Part model, mm, in its own coordinate system. A direction names the side the tool comes from. Coordinates: 2 decimals unless noted, no trailing zeros. Write each loop counter-clockwise with the first axis right and the second up, starting at its lowest first coordinate (ties: lowest second). Pieces come first, ordered by that corner, then holes. Notation, with made-up numbers: (0, 32) -> (36, 32) arc R22 cw to (36, 70) -> close; hole circle Ø9 at (-1.5, 60.25). An arc over 180 degrees is marked (long way). Write item = value, one per line. Start each with the question number.
Q1. Band-saw the part on C-C, the plane y = -6. List the corners of the cut face in (x, z), plus the area to 3 significant figures.
Q2. Tool access for faces 1 (the cylindrical face through (-1, -2, 65)), 2 (the flat face through (12, -10, 30)), 3 (the cylindrical face through (-1, -2, 15)), 4 (the cylindrical face through (13, -18, 31)): list every direction of +Z, -Z, +X, -X, +Y, -Y with a clear straight run to the whole face (end or side of a thin tool).
Q3. Pull direction Y, two halves, no side cores. Call faces 5 (the cylindrical face through (24, -18, 40)), 6 (the cylindrical face through (10, -10, 41)), 7 (the cylindrical face through (-2, -10, 1)): released by +Y, released by -Y, zero draft, split by the parting line, or undercut.
Q4. Probe line 1 (Z direction, x = 18, y = -10); line 2 (Z direction, x = 4, y = -10); line 3 (X direction, y = -7.25, z = 74.5). List the from-to ranges inside material, lowest first.
Q5. Band-saw the part on D-D, the plane x = -21. List the corners of the cut face in (y, z).
Q6. Band-saw the part on B-B, the plane z = 40. List the corners of the cut face in (x, y), plus the area to 3 significant figures.
Q7. Pin check, flat tips, straight feed: P1, Ø5, axis at x = 18.5, y = -16.5, coming from the +Z side; P2, Ø5, axis at y = -9, z = 13.5, coming from the +X side; P3, Ø6, axis at x = 10.5, z = 55, coming from the -Y side; P4, Ø11, axis at x = 15, y = -9, coming from the -Z side. Stop position of each tip, or through.
Q8. Band-saw the part on A-A, the plane x = 13. List the corners of the cut face in (y, z).
from build123d import *

# Parameters (mm, degrees)
F0_W     = 25
F0_H     = 20
F1_DEPTH = 20
F2_R     = 5
F3_R     = 1
F4_DEPTH = 30


with BuildPart() as f1:
    # F0 (on Front) → F1 (new body)
    with BuildSketch(Plane.XZ):
        Polygon((-25, 0), (0, 0), (0, 30), (0, 50), (0, 80), (-25, 80), align=None)
        with Locations((12.5, 40)):
            Rectangle(F0_W, F0_H)
    extrude(amount=F1_DEPTH)

    # F2
    f2_edges = [f1.edges().sort_by_distance(p)[0] for p in [
        (0, -20, 15),
        (25, -10, 30),
        (0, -10, 30),
        (-25, -10, 80),
        (0, -10, 80),
        (-25, -10, 0),
        (0, -20, 65),
        (0, 0, 65),
        (0, -10, 50),
        (25, -10, 50),
        (-12.5, 0, 0),
        (-12.5, -20, 0),
        (-12.5, 0, 80),
        (-12.5, -20, 80),
        (0, 0, 15),
        (-25, 0, 40),
        (-25, -20, 40),
        (12.5, 0, 30),
        (12.5, -20, 30),
        (12.5, 0, 50),
        (12.5, -20, 50),
        (0, -10, 0),
        (25, 0, 40),
        (25, -20, 40),
    ]]
    fillet(f2_edges, radius=F2_R)

    # F3 (on face) → F4 (cut)
    with BuildSketch(Plane.YZ.offset(25)):
        with Locations((-10, 40)):
            Circle(F3_R)
    extrude(amount=-F4_DEPTH, mode=Mode.SUBTRACT)


solid = f1.part
Ans:
q1.outline = (-25, 5) arc R5 ccw to (-20, 0) -> (-5, 0) arc R5 ccw to (0, 5) -> (0, 25) arc R5 cw to (5, 30) -> (20, 30) arc R5 ccw to (25, 35) -> (25, 45) arc R5 ccw to (20, 50) -> (5, 50) arc R5 cw to (0, 55) -> (0, 75) arc R5 ccw to (-5, 80) -> (-20, 80) arc R5 ccw to (-25, 75) -> close
q1.area = 2,480 mm2
q2.face_1 = +Z, +X, +Y
q2.face_2 = -Z, +X, +Y, -Y
q2.face_3 = -Z, +X, +Y
q2.face_4 = -Z, +X, -Y
q3.face_5 = released by -Y
q3.face_6 = undercut
q3.face_7 = zero draft
q4.line_1 = 30 to 39, 41 to 50
q4.line_2 = 29.9 to 39, 41 to 50.1
q4.line_3 = -25 to 0
q5.outline = (-19.9, 5) arc R4.9 ccw to (-15, 0.1) -> (-5, 0.1) arc R4.9 ccw to (-0.1, 5) -> (-0.1, 75) arc R4.9 ccw to (-5, 79.9) -> (-15, 79.9) arc R4.9 ccw to (-19.9, 75) -> close
q6.outline = (-25, -15) arc R5 ccw to (-20, -20) -> (20, -20) arc R5 ccw to (25, -15) -> (25, -11) -> (-5, -11) -> (-5, -9) -> (25, -9) -> (25, -5) arc R5 ccw to (20, 0) -> (-20, 0) arc R5 ccw to (-25, -5) -> close
q6.area = 919 mm2
q7.P1 = 50
q7.P2 = 0
q7.P3 = through
q7.P4 = 30
q8.outline = (-20, 35) arc R5 ccw to (-15, 30) -> (-5, 30) arc R5 ccw to (0, 35) -> (0, 45) arc R5 ccw to (-5, 50) -> (-15, 50) arc R5 ccw to (-20, 45) -> close; hole circle Ø2 at (-10, 40)
